from build123d import *

# Parameters (mm, degrees)
F1_DEPTH    = 8
F3_D        = 4.1
F3_DEPTH    = 7
F3_TIP      = 1.231764269
F4_W        = 43
F4_H        = 8
F5_DEPTH    = 5
F6_T        = 5
F6_T3_DEPTH = 18
F7_D        = 2.8
F7_DEPTH    = 7
F7_TIP      = 0.8412048666


# Not quite as in the source:
# - a shell that OpenCascade refuses in one call is made with other operations: the cavity is built on its own and cut out


with BuildPart() as f1:
    # F0 (on Top) → F1 (new body)
    with BuildSketch(Plane.XY):
        Polygon((22.2267507434, 11.7376726019), (-0.8732492566, 11.7376726019), (-0.8732492566, 6.7376726019), (19.2267507434, 6.7376726019), (19.2267507434, -53.2623273981), (87.2267507434, -53.2623273981), align=None)
    extrude(amount=F1_DEPTH)

    # F3
    with Locations(Plane.XZ.offset(-6.7376726019)):
        with Locations((9.1767507434, 4)):
            Hole(F3_D / 2, depth=F3_DEPTH)
            with Locations((0, 0, -(F3_DEPTH + F3_TIP / 2))):  # 118° drill point
                Cone(0, F3_D / 2, F3_TIP, mode=Mode.SUBTRACT)

    # F4 (on face) → F5 (cut)
    with BuildSketch(Plane(origin=(16.9822116726, 16.9822116726, 0), x_dir=(-0.7071067812, 0.7071067812, 0), z_dir=(0.7071067812, 0.7071067812, 0))):
        with Locations((-52.4168982823, 4)):
            Rectangle(F4_W, F4_H)
    extrude(amount=-F5_DEPTH, mode=Mode.SUBTRACT)

    # F6: shell of thickness 5, made by hand


with BuildPart() as f6_core1:
    # F6_t2: copy of F1
    add(f1.part)

    # the walls: a layer under each face that stays
    f6_faces = [f6_core1.faces().sort_by_distance(p)[0] for p in [
        (18.3767507434, 11.7376726019, 6.6666666667),
        (30.5352554223, 3.4291679229, 4),
        (-0.8732492566, 9.2376726019, 4),
        (7.1267507434, 9.2376726019, 4),
        (37.0759931483, -6.647103709, 4),
        (50.5110219908, -23.6176664575, 4),
        (67.4815847393, -37.0526953, 4),
        (78.2380512178, -44.2736278726, 4),
        (53.2267507434, -53.2623273981, 4),
        (19.2267507434, -23.2623273981, 4),
        (2.4767507434, 6.7376726019, 6.6666666667),
    ]]
    thicken(f6_faces, amount=-F6_T, mode=Mode.SUBTRACT)

    # F6_s4 → F6_t3 (cut)
    with BuildSketch(Plane.XY.offset(-5)):
        Polygon((35.3789368734, -8.414870662), (31.7726922894, -4.879336756), (28.2371583834, -8.414870662), (31.7726922894, -11.9504045679), align=None)
        Polygon((65.7138177863, -38.7497515749), (62.1782838804, -42.3559961589), (65.7138177863, -45.8915300648), (69.2493516923, -42.3559961589), align=None)
        Polygon((19.1767507434, 6.6876726019), (24.2267507434, 6.7376726019), (24.2267507434, 11.7376726019), (19.2267507434, 11.7376726019), align=None)
    extrude(amount=F6_T3_DEPTH, mode=Mode.SUBTRACT)


with BuildPart() as f1_1:
    add(f1.part)

    # what is left inside the walls is the cavity
    f6_cavity = [f6_core1.part.solids().sort_by_distance(p)[0] for p in [
        (49.691217, -31.286017, 0.05),
    ]]
    add(f6_cavity, mode=Mode.SUBTRACT)

    # F7
    with Locations(Plane(origin=(16.9822116726, 16.9822116726, 0), x_dir=(-0.7071067812, 0.7071067812, 0), z_dir=(0.7071067812, 0.7071067812, 0))):
        with Locations((-27.4168982823, 4), (-77.4168982823, 4)):
            Hole(F7_D / 2, depth=F7_DEPTH)
            with Locations((0, 0, -(F7_DEPTH + F7_TIP / 2))):  # 118° drill point
                Cone(0, F7_D / 2, F7_TIP, mode=Mode.SUBTRACT)


solid = f1_1.part
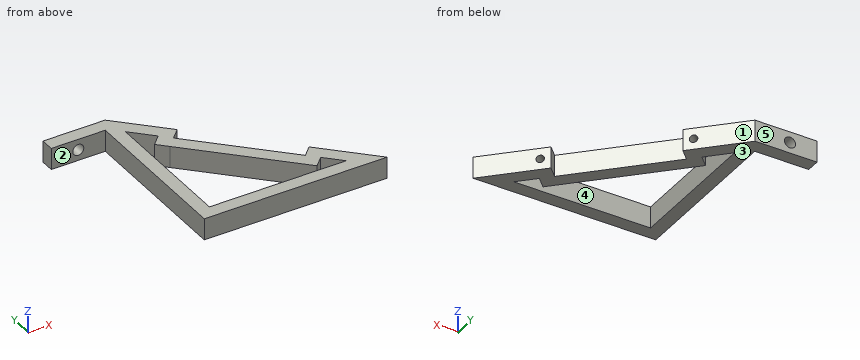
Model file for the job. Use its own axes, mm. Face numbers are marked on the shaded views. A direction names the side the tool comes from. Give positions to 0.01 mm unless a question says otherwise; leave off trailing zeros. Order: outer loops, then holes, each group sorted by start corner. A loop starts at its lowest first (then second) coordinate and runs counter-clockwise, first axis right, second up. Notation, with made-up numbers: M -27,-31.75 L 3,-31.75 A36 ccw 3,3.25 Z; hole C -9,50.25 d7. An arc over 180 degrees is marked long. Write item = value, one per line.
Q1. Cut at C-C, the plane x = 51. List the corners of the cut face in (y, z).
Derived:
outline = M -53.26,0 L -48.26,0 L -48.26,8 L -53.26,8 Z; M -31.18,0 L -24.11,0 L -24.11,8 L -31.18,8 Z
Q2. Two-plate mould, pull along Y, no slides. Class the marked faces 3, 4 and 5: pulls with the +Y half, pulls with the -Y half, needs draft (parallel to the pull), parting line crosses it, or undercut.
Derived:
face_3 = needs draft
face_4 = undercut
face_5 = pulls with the +Y half
Q3. Cut at B-B, the plane y = -14.5. List the corners of the cut face in (x, z), then the cut area to 3 significant figures.
Derived:
outline = M 19.23,0 L 24.23,0 L 24.23,8 L 19.23,8 Z; M 34.32,0 L 41.39,0 L 41.39,8 L 34.32,8 Z
area = 96.6 mm2
Q4. Tool access for the marked faces 1 and 2: list every direction of +Z, -Z, +X, -X, +Y, -Y with a clear straight run to the whole face (end or side of a thin tool).
Derived:
face_1 = +Z, -Z, +X, +Y
face_2 = +Z, -Z, -X, -Y
Q5. Drill centre lines: line 1 (Y direction, x = 35.5, z = 7); line 2 (Y direction, x = 16, z = 4); line 3 (Y direction, x = 30.5, z = 6.75). Where is each one in solid material? Low to high. Write a range as [from, to].
Derived:
line_1 = [-53.26, -48.26], [-15.68, -8.61], [-8.22, -1.54]
line_2 = [6.74, 11.74]
line_3 = [-53.26, -48.26], [-10.68, -6.15], [-3.61, 3.46]
Q6. Cut at A-A, the plane z = 7. List the corners of the cut face in (x, y), then the cut area to 3 significant figures.
Derived:
outline = M -0.87,6.74 L 19.23,6.74 L 19.23,-53.26 L 87.23,-53.26 L 69.25,-35.28 L 65.71,-38.82 L 35.31,-8.41 L 38.84,-4.88 L 22.23,11.74 L -0.87,11.74 Z; hole M 24.23,-48.26 L 75.16,-48.26 L 69.25,-42.36 L 65.71,-45.89 L 28.24,-8.41 L 31.77,-4.88 L 24.23,2.67 Z
area = 1,160 mm2
Q7. Flat gauge pins, fed straight in: pin 1 (2.5 mm diameter, centred on x = 43, z = 3, fed in from +Y); pin 2 (1 mm diameter, centred on y = -18, z = 1.5, fed in from -X); pin 3 (4 mm diameter, centred on y = -21.5, z = 2, fed in from +X). Where does each tip first touch, or does it go through?
Derived:
pin_1 = -14.86
pin_2 = 19.23
pin_3 = 50.39
Q8. Cut at D-D, the plane x = 16. List the corners of the cut face in (y, z).
Derived:
outline = M 6.74,0 L 11.74,0 L 11.74,8 L 6.74,8 Z
